```python
from build123d import *

# Parameters (mm, degrees)
F1_DEPTH = 12.7
F2_R     = 3.175
F3_DEPTH = 25.4


with BuildPart() as f1:
    # F0 (on Right) → F1 (new body)
    with BuildSketch(Plane.YZ):
        with BuildLine():
            Line((-3.82134, 0), (0, 0))
            Line((0, 0), (50.8, 0))
            Line((50.8, 0), (57.15, 0))
            Line((57.15, 0), (57.15, 19.05))
            Line((57.15, 19.05), (50.8, 19.05))
            Line((50.8, 19.05), (50.8, 6.35))
            Line((50.8, 6.35), (22.854816, 6.35))
            Line((22.854816, 6.35), (25.589257, 15.422352))
            ThreePointArc((25.589257, 15.422352), (15.227977, 13.574267), (7.574122, 6.35))
            Line((7.574122, 6.35), (0, 6.35))
            ThreePointArc((0, 6.35), (-2.73009, 3.668115), (-3.82134, 0))
        make_face()
    extrude(amount=F1_DEPTH)

    # F2 (on face) → F3 (cut)
    with BuildSketch(Plane.XZ.offset(-50.8)):
        with Locations((6.35, 12.7)):
            Circle(F2_R)
    extrude(amount=-F3_DEPTH, mode=Mode.SUBTRACT)


solid = f1.part
```
Build history of the part. All positions in model axes, mm. A direction names the side the tool comes from. Round coordinates to 2 decimals unless told otherwise and drop trailing zeros. Write each loop counter-clockwise with the first axis right and the second up, starting at its lowest first coordinate (ties: lowest second). Pieces come first, ordered by that corner, then holes. Notation, with made-up numbers: (23.25, 85.5) - (79.25, 85.5) arc R13 ccw to (79.25, 90.5) - close; hole circle Ø8 at (49.25, 61). An arc over 180 degrees is marked (long way). Answer as CSV lines item,"result".
Q1. Pull direction X, two halves, no side cores. Call faces 1 (the cylindrical face through (6.26, 15.36, 13.64)), 2 (the cylindrical face through (3.83, 53.93, 10.77)), 3 (the flat face through (0, 26, 5)): +X half, -X half, draft (parallel to the pull), parting line (faces both ways), or undercut.
Report:
face 1,"draft"
face 2,"undercut"
face 3,"-X half"
Q2. Drill centre lines: probe 1 along Z at (x, y) = (6.35, 53.75) (3 decimals); probe 2 along Z at (x, y) = (9.5, 39.5); probe 3 along Y at (x, z) = (7.75, 17). Where is each one in solid material? Low to high. Write a range as [from, to].
Report:
probe 1,"z = [0, 9.525], [15.875, 19.05]"
probe 2,"z = [0, 6.35]"
probe 3,"y = [50.8, 57.15]"
Q3. Tool access for faces 4 (the flat face through (6, 26, 0)), 5 (the flat face through (6, 4, 6.35)), 6 (the flat face through (6.261, 24.203, 10.823)), 7 (the flat face through (3, 50.8, 14)): list every direction of +Z, -Z, +X, -X, +Y, -Y with a clear straight run to the whole face (end or side of a thin tool).
Report:
face 4,"-Z, +X, -X, +Y, -Y"
face 5,"+Z, +X, -X, -Y"
face 6,"+X, -X"
face 7,"+Z, +X, -X"
Q4. Drop flat-ended pins along their axis: pin 1 (1.5 mm diameter, centred on x = 9.5, y = 6, fed in from +Z); pin 2 (5 mm diameter, centred on x = 7.5, z = 15, fed in from -Y); pin 3 (5 mm diameter, centred on x = 6.35, z = 12.7, fed in from +Y). Give the stop position or say it passes through.
Report:
pin 1,"stops at z = 6.35"
pin 2,"stops at y = 13.37"
pin 3,"stops at y = 25.52"
Q5. Cut at D-D (x = 2.5). Write the cut outline in (y, z) (3 decimals), and give its area (3 significant figures).
Report:
outline,"(-3.821, 0) - (57.15, 0) - (57.15, 19.05) - (50.8, 19.05) - (50.8, 6.35) - (22.855, 6.35) - (25.589, 15.422) arc R18.402 ccw to (7.574, 6.35) - (0, 6.35) arc R7.657 ccw to start"
area,"571 mm^2"
Q6. Cut at A-A (x = 6.35). Write the cut outline in (y, z) (3 decimals).
Report:
outline,"(-3.821, 0) - (57.15, 0) - (57.15, 9.525) - (50.8, 9.525) - (50.8, 6.35) - (22.855, 6.35) - (25.589, 15.422) arc R18.402 ccw to (7.574, 6.35) - (0, 6.35) arc R7.657 ccw to start; (50.8, 15.875) - (57.15, 15.875) - (57.15, 19.05) - (50.8, 19.05) - close"
Q7. Cut at C-C (y = 23.5). Write the cut outline in (x, z), and give its area (3 significant figures).
Report:
outline,"(0, 0) - (12.7, 0) - (12.7, 6.35) - (0, 6.35) - close; (0, 8.49) - (12.7, 8.49) - (12.7, 15.54) - (0, 15.54) - close"
area,"170 mm^2"
Q8. Cut at B-B (z = 10.75). Write the cut outline in (x, y), and give its area (3 significant figures).
Report:
outline,"(0, 11.12) - (12.7, 11.12) - (12.7, 24.18) - (0, 24.18) - close; (0, 50.8) - (3.84, 50.8) - (3.84, 57.15) - (0, 57.15) - close; (8.86, 50.8) - (12.7, 50.8) - (12.7, 57.15) - (8.86, 57.15) - close"
area,"215 mm^2"
